For this review, take the finished solid that the model builds, in its own axes (mm). Round coordinates to 2 decimals unless told otherwise and drop trailing zeros. Write each loop counter-clockwise with the first axis right and the second up, starting at its lowest first coordinate (ties: lowest second). Pieces come first, ordered by that corner, then holes. Notation, with made-up numbers: (64, 15) -> (75, 15) arc R26 ccw to (75, 50) -> close; hole circle Ø2 at (47, 62.5). An arc over 180 degrees is marked (long way). Answer in a Markdown table with one row per item. Add a question column.
```python
from build123d import *

# Parameters (mm, degrees)
F0_W     = 50.8
F0_H     = 127
F1_DEPTH = 50.544538
F2_R     = 12.7
F3_R     = 6.35
F4_DEPTH = 105.582835


with BuildPart() as f1:
    # F0 (on Top) → F1 (new body)
    with BuildSketch(Plane.XY):
        with Locations((0, 1.760196)):
            Rectangle(F0_W, F0_H)
    extrude(amount=F1_DEPTH)

    # F2
    f2_edges = [f1.edges().sort_by_distance(p)[0] for p in [
        (25.4, 1.760196, 50.544538),
        (0, -61.739804, 50.544538),
        (-25.4, 1.760196, 50.544538),
        (0, 65.260196, 50.544538),
    ]]
    fillet(f2_edges, radius=F2_R)

    # F3 (on face) → F4 (cut)
    with BuildSketch(Plane.YZ.offset(25.4)):
        with Locations((0, 12.333511)):
            Circle(F3_R)
    extrude(amount=-F4_DEPTH, mode=Mode.SUBTRACT)


solid = f1.part
```
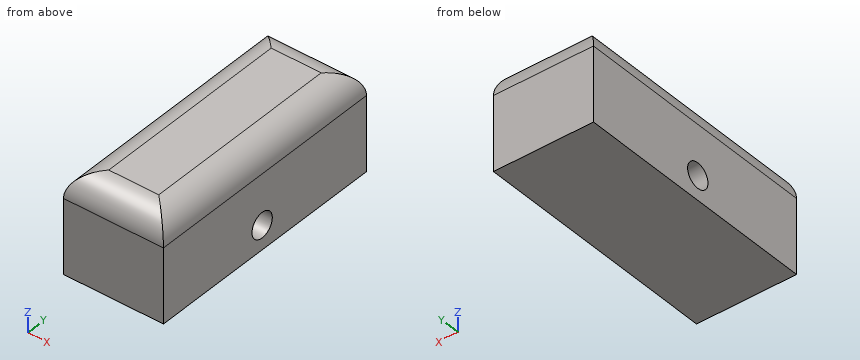
1. For L1, parallel to Y at x = -5, z = 12.5; L2, parallel to Z at x = 12, y = 0; L3, parallel to Y at x = -3, z = 9, list the stretches that pass through material, from the lowest coordinate up. Write a range as [from, to].
2. We need section A-A (y = 0). Write out the cut boundary in (x, z), plus the area to 3 significant figures.
3. We need section D-D (x = 5). Write out the cut boundary in (y, z).
4. We need section B-B (z = 16.5). Write out the cut boundary in (x, y), plus the area to 3 significant figures.
5. We need section C-C (x = 21). Write out the cut boundary in (y, z), plus the area to 3 significant figures.
Response:
| question | item | result |
|---|---|---|
| 1 | L1 | [-61.74, -6.35], [6.35, 65.26] |
| 1 | L2 | [0, 5.98], [18.68, 50.54] |
| 1 | L3 | [-61.74, -5.4], [5.4, 65.26] |
| 2 | outline | (-25.4, 0) -> (25.4, 0) -> (25.4, 5.98) -> (-25.4, 5.98) -> close; (-25.4, 18.68) -> (25.4, 18.68) -> (25.4, 37.84) arc R12.7 ccw to (12.7, 50.54) -> (-12.7, 50.54) arc R12.7 ccw to (-25.4, 37.84) -> close |
| 2 | area | 1,850 mm2 |
| 3 | outline | (-61.74, 0) -> (65.26, 0) -> (65.26, 37.84) arc R12.7 ccw to (52.56, 50.54) -> (-49.04, 50.54) arc R12.7 ccw to (-61.74, 37.84) -> close; hole circle Ø12.7 at (0, 12.33) |
| 4 | outline | (-25.4, -61.74) -> (25.4, -61.74) -> (25.4, -4.79) -> (-25.4, -4.79) -> close; (-25.4, 4.79) -> (25.4, 4.79) -> (25.4, 65.26) -> (-25.4, 65.26) -> close |
| 4 | area | 5,960 mm2 |
| 5 | outline | (-61.74, 0) -> (65.26, 0) -> (65.26, 37.84) arc R12.7 ccw to (60.86, 47.46) -> (-57.34, 47.46) arc R12.7 ccw to (-61.74, 37.84) -> close; hole circle Ø12.7 at (0, 12.33) |
| 5 | area | 5,870 mm2 |
